Build history of the part. All positions in model axes, mm. A direction names the side the tool comes from. Round coordinates to 2 decimals unless told otherwise and drop trailing zeros. Write each question's results on one line, items separated by ' | '. Start each with the question number.
```python
from build123d import *

# Parameters (mm, degrees)
BOSS_EXTRUDE1_DEPTH = 10
SKETCH3_W           = 210
SKETCH3_H           = 10
BOSS_EXTRUDE2_DEPTH = 10
SKETCH4_R           = 1
CUT_EXTRUDE1_DEPTH  = 10


with BuildPart() as part:
    # Sketch1 → Boss-Extrude1 (new body)
    with BuildSketch(Plane(origin=(0, 0, 0), x_dir=(-1, 0, 0), z_dir=(0, 0, -1))):
        Polygon((-105, -1.902946103), (-105, -8), (105, -8), (105, -3.75), (103.017387777, -3.75), (100.560588695, 3), (98.032021121, 3), (95.575222039, -3.75), (93.592609816, -3.75), (91.135810735, 3), (88.60724316, 3), (86.150444078, -3.75), (84.167831855, -3.75), (81.711032774, 3), (79.182465199, 3), (76.725666118, -3.75), (74.743053894, -3.75), (72.286254813, 3), (69.757687238, 3), (67.300888157, -3.75), (65.318275934, -3.75), (62.861476852, 3), (60.332909277, 3), (57.876110196, -3.75), (55.893497973, -3.75), (53.436698891, 3), (50.908131317, 3), (48.451332235, -3.75), (46.468720012, -3.75), (44.011920931, 3), (41.483353356, 3), (39.026554275, -3.75), (37.043942051, -3.75), (34.58714297, 3), (32.058575395, 3), (29.601776314, -3.75), (27.61916409, -3.75), (25.162365009, 3), (22.633797434, 3), (20.176998353, -3.75), (18.19438613, -3.75), (15.737587048, 3), (13.209019474, 3), (10.752220392, -3.75), (8.769608169, -3.75), (6.312809088, 3), (3.784241513, 3), (1.327442432, -3.75), (-0.655169792, -3.75), (-3.111968873, 3), (-5.640536448, 3), (-8.097335529, -3.75), (-10.079947753, -3.75), (-12.536746834, 3), (-15.065314409, 3), (-17.52211349, -3.75), (-19.504725713, -3.75), (-21.961524795, 3), (-24.490092369, 3), (-26.946891451, -3.75), (-28.929503674, -3.75), (-31.386302755, 3), (-33.91487033, 3), (-36.371669412, -3.75), (-38.354281635, -3.75), (-40.811080716, 3), (-43.339648291, 3), (-45.796447372, -3.75), (-47.779059596, -3.75), (-50.235858677, 3), (-52.764426252, 3), (-55.221225333, -3.75), (-57.203837556, -3.75), (-59.660636638, 3), (-62.189204213, 3), (-64.646003294, -3.75), (-66.628615517, -3.75), (-69.085414599, 3), (-71.613982173, 3), (-74.070781255, -3.75), (-76.053393478, -3.75), (-78.510192559, 3), (-81.038760134, 3), (-83.495559215, -3.75), (-85.478171439, -3.75), (-87.93497052, 3), (-90.463538095, 3), (-92.920337176, -3.75), (-94.9029494, -3.75), (-97.359748481, 3), (-99.888316056, 3), (-102.345115137, -3.75), (-104.32772736, -3.75), align=None)
    extrude(amount=-BOSS_EXTRUDE1_DEPTH)

    # Sketch3 → Boss-Extrude2 (add)
    with BuildSketch(Plane.XZ.offset(8)):
        with Locations((0, 5)):
            Rectangle(SKETCH3_W, SKETCH3_H)
    extrude(amount=BOSS_EXTRUDE2_DEPTH)

    # Sketch4 → Cut-Extrude1 (cut)
    with BuildSketch(Plane.ZY.offset(105)):
        with Locations((5, -10.9)):
            Circle(SKETCH4_R)
    extrude(amount=-CUT_EXTRUDE1_DEPTH, mode=Mode.SUBTRACT)


solid = part.part
```
1. Flat gauge pins, fed straight in: pin 1 Ø0.6 at (x, z) = (-94.5, 3.5) entering from +Y; pin 2 Ø6 at (y, z) = (0, 3.5) entering from -X. Where does each tip first touch, or does it go through?
2. Mould opens along X. For faces 1 (the face through (105, -10, 5)), 2 (the face through (-1, -18, 5)), 3 (the face through (-7.558, -0.422, 4.93)) say: pulls with the +X half, pulls with the -X half, needs draft (parallel to the pull), parting line crosses it, or undercut.
3. 3-axis set-ups, long thin cutter, end or side, ignore diameter. For faces 4 (the face through (-2.573, -0.328, 4.93)), 5 (the face through (-1, -10, 10)): which of +Z, -Z, +X, -X, +Y, -Y reach the whole face in a straight line?
4. Wall check: line 1 (Y direction, x = 93, z = 7); line 2 (Y direction, x = -99.5, z = 5); line 3 (Z direction, x = -96, y = -10). Give the ranges that are in metal, low to high. Write a range as from..to.
A:
1) pin 1: stops at y = -3.75 | pin 2: stops at x = -102.74
2) face 1: pulls with the +X half | face 2: needs draft | face 3: undercut
3) face 4: +Z, -Z, +Y | face 5: +Z, +X, -X, +Y, -Y
4) line 1: y = -18..-3.75 | line 2: y = -18..-11.9, -9.9..3 | line 3: z = 0..4.56, 5.44..10
